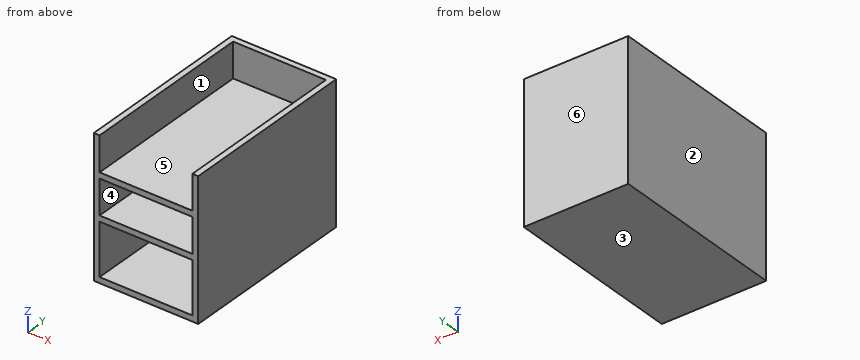
from build123d import *

# Parameters (mm, degrees)
F0_W      = 203.2
F0_H      = 381
F1_DEPTH  = 12.7
F2_W      = 203.2
F2_H      = 292.1
F2_H_2    = 12.7
F3_DEPTH  = 12.7
F4_W      = 381
F4_H      = 292.1
F5_DEPTH  = 12.7
F6_W      = 381
F6_H      = 292.1
F7_DEPTH  = 12.7
F8_W      = 203.2
F8_H      = 12.7
F9_DEPTH  = 381
F10_W     = 203.2
F10_H     = 12.7
F11_DEPTH = 381


with BuildPart() as f1:
    # F0 (on Top) → F1 (new body)
    with BuildSketch(Plane.XY):
        Rectangle(F0_W, F0_H)
    extrude(amount=F1_DEPTH)

    # F2 (on face) → F3 (join)
    with BuildSketch(Plane(origin=(0, 190.5, 0), x_dir=(-1, 0, 0), z_dir=(0, 1, 0))):
        with Locations((0, 158.75)):
            Rectangle(F2_W, F2_H)
        with Locations((0, 6.35)):
            Rectangle(F2_W, F2_H_2)
    extrude(amount=F3_DEPTH)

    # F4 (on face) → F5 (join)
    with BuildSketch(Plane.YZ.offset(101.6)):
        with Locations((0, 158.75)):
            Rectangle(F4_W, F4_H)
        Polygon((-190.5, 0), (203.2, 0), (203.2, 304.8), (190.5, 304.8), (190.5, 12.7), (-190.5, 12.7), align=None)
    extrude(amount=F5_DEPTH)

    # F6 (on face) → F7 (join)
    with BuildSketch(Plane(origin=(-101.6, 0, 0), x_dir=(0, -1, 0), z_dir=(-1, 0, 0))):
        Polygon((-203.2, 304.8), (-203.2, 0), (190.5, 0), (190.5, 12.7), (-190.5, 12.7), (-190.5, 304.8), align=None)
        with Locations((0, 158.75)):
            Rectangle(F6_W, F6_H)
    extrude(amount=F7_DEPTH)

    # F8 (on face) → F9 (join)
    with BuildSketch(Plane.XZ.offset(-190.5)):
        with Locations((0, 222.25)):
            Rectangle(F8_W, F8_H)
    extrude(amount=F9_DEPTH)

    # F10 (on face) → F11 (join)
    with BuildSketch(Plane.XZ.offset(-190.5)):
        with Locations((0, 133.35)):
            Rectangle(F10_W, F10_H)
    extrude(amount=F11_DEPTH)


solid = f1.part
Here's how the part is built. I have some questions about the finished solid (model axes, mm). Face numbers are marked on the shaded views. A direction names the side the tool comes from. Coordinates: 2 decimals unless noted, no trailing zeros. Loops run counter-clockwise (first coordinate to the right, second up) from the corner with the lowest first, then second, coordinate; pieces in that order, holes last. Notation, with made-up numbers: (26.5, -18.75) -> (34.5, -18.75) arc R18 ccw to (34.5, -8.75) -> close; hole circle Ø2 at (75, -39.5). An arc over 180 degrees is marked (long way). Use one line per item in the form item = value. Start each with the question number.
(1) If we section it at A-A (y = -98): Please give me the cut outline in (x, z), then the cut area to 3 significant figures.
(2) If we section it at B-B (z = 255): Please give me the cut outline in (x, y), then the cut area to 3 significant figures.
(3) If we section it at C-C (x = -39.5): Please give me the cut outline in (y, z).
(4) Please list where these lines run through material, in increasing order: line 1 along Z through (x, y) = (-32, 130); line 2 along X through (y, z) = (-122.5, 82); line 3 along Y through (x, z) = (44, 170).
(5) Will these pins go through, and if not, where does the flat tip stop? pin 1 (4 mm diameter, centred on x = 89, y = -32, fed in from +Z); pin 2 (1.5 mm diameter, centred on x = -38.5, z = 171, fed in from -Y).
(6) On a 3-axis mill with a long thin cutter (end or side, diameter ignored), from which of +Z, -Z, +X, -X, +Y, -Y can I reach the whole of each face in a straight line? I mean the marked faces 4, 5 and 6. Say none if no direction works.
(7) We'd pull the mould along X, two halves only. Please class the marked faces 1, 2 and 3: pulls with the +X half, pulls with the -X half, needs draft (parallel to the pull), parting line crosses it, or undercut.
Verdict:
q1.outline = (-114.3, 0) -> (114.3, 0) -> (114.3, 304.8) -> (101.6, 304.8) -> (101.6, 228.6) -> (-101.6, 228.6) -> (-101.6, 304.8) -> (-114.3, 304.8) -> close; hole (-101.6, 12.7) -> (101.6, 12.7) -> (101.6, 127) -> (-101.6, 127) -> close; hole (-101.6, 139.7) -> (101.6, 139.7) -> (101.6, 215.9) -> (-101.6, 215.9) -> close
q1.area = 15,500 mm²
q2.outline = (-114.3, -190.5) -> (-101.6, -190.5) -> (-101.6, 190.5) -> (101.6, 190.5) -> (101.6, -190.5) -> (114.3, -190.5) -> (114.3, 203.2) -> (-114.3, 203.2) -> close
q2.area = 12,600 mm²
q3.outline = (-190.5, 0) -> (203.2, 0) -> (203.2, 304.8) -> (190.5, 304.8) -> (190.5, 228.6) -> (-190.5, 228.6) -> (-190.5, 215.9) -> (190.5, 215.9) -> (190.5, 139.7) -> (-190.5, 139.7) -> (-190.5, 127) -> (190.5, 127) -> (190.5, 12.7) -> (-190.5, 12.7) -> close
q4.line_1 = 0 to 12.7, 127 to 139.7, 215.9 to 228.6
q4.line_2 = -114.3 to -101.6, 101.6 to 114.3
q4.line_3 = 190.5 to 203.2
q5.pin_1 = 228.6
q5.pin_2 = 190.5
q6.face_4 = -Y
q6.face_5 = +Z, -Y
q6.face_6 = +Z, -Z, +X, -X, +Y
q7.face_1 = undercut
q7.face_2 = pulls with the -X half
q7.face_3 = needs draft
